Geometry: final body of the model. Coordinates: model frame, mm. Coordinates: 2 decimals unless noted, no trailing zeros. Order: outer loops, then holes, each group sorted by start corner. A loop starts at its lowest first (then second) coordinate and runs counter-clockwise, first axis right, second up. Notation, with made-up numbers: M 33.25,-23.5 L 84.25,-23.5 A14 cw 84.25,-4.5 Z; hole C 3,10 d2. An arc over 180 degrees is marked long. Write item = value, one per line.
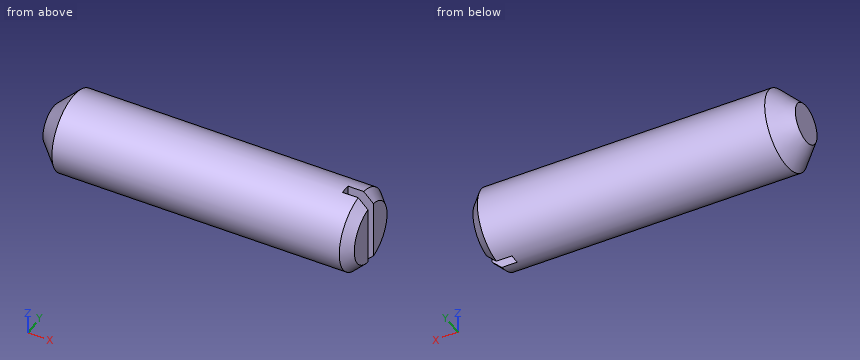
Autodesk Inventor part; units mm, degrees
ref_plane "Work Plane1" through (4, 0, 0) normal (0, 0, 1) x (1, 0, 0)
ref_plane "YZ Plane" through (0, 0, 0) normal (1, 0, 0) x (0, 1, 0)
ref_plane "XZ Plane" through (0, 0, 0) normal (0, 1, 0) x (-1, 0, 0)
sketch "Sketch1" plane through (0, 0, 0) normal (0, 0, 1) x (1, 0, 0)
  line L0 (0, 0) -> (8, 0)
  line L1 (8, 0) -> (8, 1)
  line L2 (8, 1) -> (0, 1)
  line L3 (0, -0.2) -> (0, 1.2)
  line L4 (0, 1) -> (0, 0)
  dimension "d0" = 2
  dimension "d2" = 8
revolve "Body" add sketch "Sketch1" angle 360 about axis through (0, 0, 0) along (1, 0, 0)
chamfer "Chamfer1" distance 0.2454 angle 45 1 edges at (8, -1, 0) measured on face at (8, 0.3808, -0.3117)
sketch "Sketch2" plane through (0, 0, 0) normal (0, 0, 1) x (1, 0, 0)
  line L0 (8, 0.7546) -> (8, -0.7546)
  line L1 (7.232, 0) -> (8.128, 0)
  line L2 (8, 0.125) -> (7.36, 0.125)
  line L3 (7.36, 0.125) -> (7.36, 0)
  line L4 (7.36, -0.125) -> (7.36, 0)
  line L5 (7.36, -0.125) -> (8, -0.125)
  dimension "d8" = 0.125
  dimension "d9" = 0.64
extrude "Slot1" cut sketch "Sketch2" against normal mid plane 2
thread "Thread"
chamfer "Chamfer2" distance 0.5 angle 45 1 edges at (0, -1, 0) measured on face at (2.5849, -0.4298, 0.9029)
ref_plane "Work Plane1" through (4, 0, 0) normal (0, 0, 1) x (1, 0, 0)
equation "\"d8\" = 0.5 * SBR"
equation "\"d9\" = STI"
equation "\"d10\" = NND"
equation "\"d3\" = -0.5 * GD1 + 0.5 * NND"
equation "\"d4\" = FAWI"
equation "\"d34\" = -0.5 * GD1 + 0.5 * NND"
equation "\"d5\" = NLG"
equation "\"d14\" = FAWI"
equation "\"d0\" = NND"
equation "\"d2\" = NLG"
equation "\"NND\" = 2"
equation "\"NLG\" = 8"
equation "\"FAWI\" = 45deg"
equation "\"GD1\" = THREADDIA - 1.2269 * PTC"
equation "\"FAWI1\" = 45deg"
equation "\"SPD\" = 1"
equation "\"SBR\" = 0.25"
equation "\"STI\" = 0.64"
equation "\"GUL\" = 0.61345 * PTC"
equation "\"THREADDIA\" = 2"
equation "\"TOA\" = 30deg"
equation "\"PTC\" = 0.4"
equation "\"GAL\" = 0.61345 * PTC"
properties part number "ISO 4766 - M2 x 8" material "Stainless Steel, 440C"
1) Section C-C, the plane x = 1. Return loops of the section in (y, z).
Numbers:
outline = C 0,0 d2
2) Pin query (flat end, axial travel): pin 1 (0.7 mm diameter, centred on x = 7.5, z = 0.5, fed in from -Y). Return the tip coordinate at first contact, or that it passes through.
Numbers:
pin_1 = -0.99
3) Line query: L1, parallel to Z at x = 1.5, y = 0.05; L2, parallel to X at y = -0.05, z = -0.45; L3, parallel to Y at x = 7.5, z = -0.25 (3 decimals). Output: solid intervals per line, ascending.
Numbers:
L1 = -1 to 1
L2 = 0 to 7.36
L3 = -0.968 to -0.125, 0.125 to 0.968
4) Section B-B, the plane z = 0. Return loops of the section in (x, y) (3 decimals).
Numbers:
outline = M 0,-0.5 L 0.5,-1 L 7.755,-1 L 8,-0.755 L 8,-0.125 L 7.36,-0.125 L 7.36,0.125 L 8,0.125 L 8,0.755 L 7.755,1 L 0.5,1 L 0,0.5 Z
5) Section A-A, the plane y = 0. Return loops of the section in (x, z), and give its area (3 significant figures).
Numbers:
outline = M 0,-0.5 L 0.5,-1 L 7.36,-1 L 7.36,1 L 0.5,1 L 0,0.5 Z
area = 14.5 mm²
